```python
from build123d import *

# Parameters (mm, degrees)
F0_W     = 46.99
F0_H     = 18.796
F1_DEPTH = 6.096
F2_R     = 2.54
F3_W     = 46.99
F3_H     = 18.796
F3_R     = 4.445
F4_DEPTH = 3.556
F4_TAPER = -8
F5_R     = 3.175
F6_DEPTH = 2.032
F6_TAPER = -5
F7_DEPTH = 1.27


with BuildPart() as f1:
    # F0 (on Top) → F1 (new body)
    with BuildSketch(Plane.XY):
        Rectangle(F0_W, F0_H)
    extrude(amount=F1_DEPTH)

    # F2
    f2_edges = [f1.edges().sort_by_distance(p)[0] for p in [
        (-23.495, 0, 6.096),
        (23.495, 0, 6.096),
        (0, -9.398, 6.096),
        (0, 9.398, 6.096),
    ]]
    fillet(f2_edges, radius=F2_R)

    # F3 (on face) → F4 (cut)
    with BuildSketch(Plane(origin=(0, 0, 0), x_dir=(1, 0, 0), z_dir=(0, 0, -1))):
        Rectangle(F3_W, F3_H)
        Circle(F3_R, mode=Mode.SUBTRACT)
    extrude(amount=-F4_DEPTH, taper=F4_TAPER, mode=Mode.SUBTRACT)

    # F5 (on face) → F6 (cut)
    with BuildSketch(Plane(origin=(0, 0, 0), x_dir=(1, 0, 0), z_dir=(0, 0, -1))):
        Circle(F5_R)
    extrude(amount=-F6_DEPTH, taper=F6_TAPER, mode=Mode.SUBTRACT)

    # F7 (add): a face of the model
    f7_faces = [f1.faces().sort_by_distance(p)[0] for p in [
        (22.9889022114, 0, 3.556),
    ]]
    extrude(f7_faces, amount=F7_DEPTH)


solid = f1.part
```
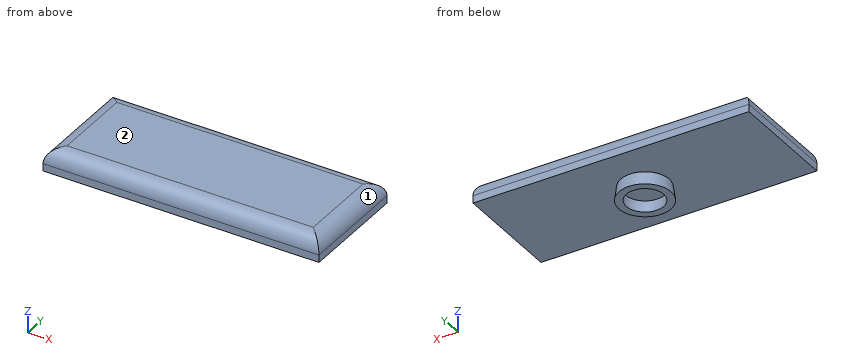
Can you work these out from the model? Positions are in its coordinate system, mm. Face numbers are marked on the shaded views. Give positions to 0.01 mm unless a question says otherwise; leave off trailing zeros. Loops run counter-clockwise (first coordinate to the right, second up) from the corner with the lowest first, then second, coordinate; pieces in that order, holes last. Notation, with made-up numbers: M 75,-20 L 85,-20 A13 cw 85,-13 Z; hole C 10,0 d3. An arc over 180 degrees is marked long. Use one line per item in the form item = value. Start each with the question number.
(1) I want a section at D-D, the plane x = 0. Write out the boundary of the cut face in (y, z) (3 decimals).
(2) I want a section at C-C, the plane z = 5.5. Write out the boundary of the cut face in (x, y).
(3) Please list where these lines run through material, in increasing order: line 1 (Z direction, x = 14.5, y = -7); line 2 (Y direction, x = 1, z = 0.5); line 3 (X direction, y = -1.25, z = 1.25).
(4) I'm going to push flat-ended pins straight in: P1, Ø1, axis at y = 0.5, z = 5, coming from the -X side; P2, Ø1, axis at x = 12.5, z = 5, coming from the +Y side. Where does each tip first touch, or does it pass through?
(5) I want a section at B-B, the plane y = 6. Write out the boundary of the cut face in (x, z) (3 decimals).
(6) Thinking about a two-plate mould opening in X: for the marked faces 1 and 2, which applies, released by +X, released by -X, zero draft, split by the parting line, or undercut?
(7) I want a section at A-A, the plane x = -20.5. Write out the boundary of the cut face in (y, z), and give its area (3 significant figures).
Worked out:
q1.outline = M -9.398,2.286 L -4.124,2.286 L -4.445,0 L -3.175,0 L -3.353,2.032 L 3.353,2.032 L 3.175,0 L 4.445,0 L 4.124,2.286 L 9.398,2.286 L 9.398,3.556 A2.54 ccw 6.858,6.096 L -6.858,6.096 A2.54 ccw -9.398,3.556 Z
q2.outline = M -22.59,-8.49 L 22.59,-8.49 L 22.59,8.49 L -22.59,8.49 Z
q3.line_1 = 2.29 to 6.09
q3.line_2 = -4.26 to -3.06, 3.06 to 4.26
q3.line_3 = -4.08 to -3.04, 3.04 to 4.08
q4.P1 = -23.31
q4.P2 = 9.22
q5.outline = M -23.495,2.286 L 23.495,2.286 L 23.495,3.556 A2.54 ccw 20.955,6.096 L -20.955,6.096 A2.54 ccw -23.495,3.556 Z
q6.face_1 = released by +X
q6.face_2 = zero draft
q7.outline = M -9.4,2.29 L 9.4,2.29 L 9.4,3.56 A2.54 ccw 6.86,6.1 L -6.86,6.1 A2.54 ccw -9.4,3.56 Z
q7.area = 68.8 mm²
